Autodesk Inventor part; units mm, degrees
ref_plane "YZ Plane" through (0, 0, 0) normal (1, 0, 0) x (0, 1, 0)
ref_plane "XZ Plane" through (0, 0, 0) normal (0, 1, 0) x (-1, 0, 0)
ref_plane "XY Plane" through (0, 0, 0) normal (0, 0, 1) x (1, 0, 0)
sketch "Sketch1" plane through (0.1451, -0.1451, 0) normal (0, 0, 1) x (1, 0, 0)
  arc A0 (20.126, -22.2473) -> (-20.126, -22.2473) centre (0, 0) ccw construction
  circle A1 centre (0, 0) radius 33 construction
  line L0 (33, 33) -> (-33, 33)
  line L1 (-33, 33) -> (-33, -33)
  line L2 (-33, -33) -> (33, -33)
  line L3 (33, -33) -> (33, 33)
  line L4 (33, 33) -> (23.3345, 23.3345) construction
  line L5 (-33, 33) -> (-23.3345, 23.3345) construction
  line L6 (23.3345, 23.3345) -> (-23.3345, -23.3345) construction
  line L7 (23.3345, -23.3345) -> (33, -33) construction
  line L8 (-23.3345, -23.3345) -> (-33, -33) construction
  line L9 (-23.3345, 23.3345) -> (23.3345, -23.3345) construction
  line L10 (0, -33) -> (0, 33) construction
  line L11 (33, 0) -> (-33, 0) construction
  circle A2 centre (0, 0) radius 1.5
  circle A3 centre (0, 0) radius 4.5
  line L12 (4.0607, -1.9393) -> (22.2473, -20.126) construction
  line L13 (1.9393, -4.0607) -> (17.8, -19.9213) construction
  arc A4 (0, -30) -> (17.8, -24.1487) centre (0, 0) ccw construction
  line L14 (-1.9393, -4.0607) -> (-17.8, -19.9213) construction
  line L15 (-4.0607, -1.9393) -> (-22.2473, -20.126) construction
  line L16 (23.3345, 23.3345) -> (-23.3345, -23.3345) construction
  arc A5 (-20.126, -22.2473) -> (-17.8, -24.1487) centre (0, 0) ccw construction
  line L17 (17.8, -24.1487) -> (17.8, -19.9213) construction
  line L18 (-17.8, -24.1487) -> (-17.8, -19.9213) construction
  line L19 (17.8, -22.035) -> (-17.8, -22.035) construction
  arc A6 (-17.8, -24.1487) -> (0, -30) centre (0, 0) ccw construction
  line L20 (-17.8, -19.9213) -> (-20.126, -22.2473) construction
  line L21 (17.8, -19.9213) -> (20.126, -22.2473) construction
  arc A7 (17.8, -24.1487) -> (20.126, -22.2473) centre (0, 0) ccw construction
  line L22 (17.8, 19.9213) -> (20.126, 22.2473) construction
  arc A8 (20.126, 22.2473) -> (17.8, 24.1487) centre (0, 0) ccw construction
  arc A9 (-17.8, 24.1487) -> (-20.126, 22.2473) centre (0, 0) ccw construction
  line L23 (-17.8, 19.9213) -> (-20.126, 22.2473) construction
  line L24 (-1.9393, 4.0607) -> (-17.8, 19.9213)
  line L25 (1.9393, 4.0607) -> (17.8, 19.9213)
  line L26 (17.8, 24.1487) -> (17.8, 19.9213)
  arc A10 (17.8, 24.1487) -> (0, 30) centre (0, 0) ccw
  arc A11 (0, 30) -> (-17.8, 24.1487) centre (0, 0) ccw
  line L27 (-17.8, 24.1487) -> (-17.8, 19.9213)
  circle A12 centre (28.1673, -28.1673) radius 2.55
  circle A13 centre (-28.1673, -28.1673) radius 2.55
  circle A14 centre (-28.1673, 28.1673) radius 2.55
  circle A15 centre (28.1673, 28.1673) radius 2.55
  point P0 (0, -22.035)
  dimension "d17" = 60
  dimension "d18" = 3
  dimension "d19" = 3
  dimension "d20" = 3
  dimension "d21" = 1.5
  dimension "d22" = 3
  dimension "d23" = 35.6
  dimension "d24" = 5.1
  dimension "d25" = 5.1
  dimension "d26" = 5.1
  dimension "d27" = 5.1
extrude "Extrusion1" add sketch "Sketch1" along normal blind 2 contours L3 L2 L1 L0 | A3
fillet "Fillet3" radius 2 10 edges at (17.9451, 24.0036, 1) (17.9451, 19.7762, 1) (33.1451, 32.8549, 1) (-32.8549, 32.8549, 1) (2.0845, 3.9155, 1) (-1.7942, 3.9155, 1) (-17.6549, 24.0036, 1) (-17.6549, 19.7762, 1) (33.1451, -33.1451, 1) (-32.8549, -33.1451, 1)
ref_plane "Work Plane4" through (-30.8549, -0.1451, 0) normal (0, -1, 0) x (1, 0, 0)
ref_plane "Work Plane5" through (0.1451, -31.1451, 0) normal (1, 0, 0) x (0, 0, -1)
properties part number "Feeder Top Plate" material "Aluminum 6061"
Model file for the job. Use its own axes, mm. A direction names the side the tool comes from. Coordinates: 2 decimals unless noted, no trailing zeros. Order: outer loops, then holes, each group sorted by start corner. A loop starts at its lowest first (then second) coordinate and runs counter-clockwise, first axis right, second up. Notation, with made-up numbers: M -17.5,82 L -10.5,82 A13 cw -10.5,92 Z; hole C 67.5,74.5 d1. An arc over 180 degrees is marked long. Return JSON: item names as keys, results as strings.
1. Pull direction X, two halves, no side cores. Call faces 1 (the face through (32.544, -32.575, 1.014)), 2 (the face through (-17.507, 19.849, 1.014)), 3 (the face through (-9.77, 11.89, 0.99)), 4 (the face through (-32.253, 32.285, 1.014)): +X half, -X half, draft (parallel to the pull), parting line (faces both ways), or undercut.
Ans:
{"face 1": "+X half", "face 2": "undercut", "face 3": "undercut", "face 4": "-X half"}
2. Saw through at C-C (z = 1.65). Give the cut face in (x, y), and give its area (3 significant figures).
Ans:
{"outline": "M -32.85,-31.15 A2 ccw -30.85,-33.15 L 31.15,-33.15 A2 ccw 33.15,-31.15 L 33.15,30.85 A2 ccw 31.15,32.85 L -30.85,32.85 A2 ccw -32.85,30.85 Z; hole C -28.02,-28.31 d5.1; hole C -28.02,28.02 d5.1; hole M -17.65,20.6 A2 ccw -17.07,19.19 L -2.67,4.79 A2 ccw -0.82,4.25 A4.5 cw 1.11,4.25 A2 ccw 2.96,4.79 L 17.36,19.19 A2 ccw 17.95,20.6 L 17.95,22.97 A2 ccw 17.07,24.62 A30 ccw 0.15,29.85 A30 ccw -16.78,24.62 A2 ccw -17.65,22.97 Z; hole C 0.15,-0.15 d3; hole C 28.31,-28.31 d5.1; hole C 28.31,28.02 d5.1", "area": "3,660 mm^2"}
3. Saw through at A-A (y = 27). Give the cut face in (x, z).
Ans:
{"outline": "M -32.85,0 L -30.36,0 L -30.36,2 L -32.85,2 Z; M -25.69,0 L -12.63,0 L -12.63,2 L -25.69,2 Z; M 12.92,0 L 25.98,0 L 25.98,2 L 12.92,2 Z; M 30.65,0 L 33.15,0 L 33.15,2 L 30.65,2 Z"}
4. Tool access for faces 5 (the face through (-17.655, 22, 1)), 6 (the face through (32.575, 32.253, 1.014)): list every direction of +Z, -Z, +X, -X, +Y, -Y with a clear straight run to the whole face (end or side of a thin tool).
Ans:
{"face 5": "+Z, -Z", "face 6": "+Z, -Z, +X, +Y"}
5. Saw through at D-D (x = -10). Give the cut face in (y, z), and give its area (3 significant figures).
Ans:
{"outline": "M -33.15,0 L 12.12,0 L 12.12,2 L -33.15,2 Z; M 28.09,0 L 32.85,0 L 32.85,2 L 28.09,2 Z", "area": "100 mm^2"}
6. Drill centre lines: probe 1 along X at (y, z) = (21, 0.95); probe 2 along Y at (x, z) = (-26.5, 1.4); probe 3 along Y at (x, z) = (-27, 1.35). Where is each one in solid material? Low to high.
Ans:
{"probe 1": "-32.85 to -17.65, 17.95 to 33.15", "probe 2": "-33.15 to -30.36, -26.27 to 25.98, 30.07 to 32.85", "probe 3": "-33.15 to -30.65, -25.98 to 25.69, 30.36 to 32.85"}
7. Saw through at B-B (x = -28.5). Give the cut face in (y, z), and give its area (3 significant figures).
Ans:
{"outline": "M -33.15,0 L -30.82,0 L -30.82,2 L -33.15,2 Z; M -25.81,0 L 25.52,0 L 25.52,2 L -25.81,2 Z; M 30.53,0 L 32.85,0 L 32.85,2 L 30.53,2 Z", "area": "112 mm^2"}
